The drawing under review shows one solid part. Ordinate dimensions are in mm from its lowest x, y, z. A direction names the side the tool comes from. Coordinates: 2 decimals unless noted, no trailing zeros. Write each loop counter-clockwise with the first axis right and the second up, starting at its lowest first coordinate (ties: lowest second). Pieces come first, ordered by that corner, then holes.
1) For P1, Ø2, axis at x = 31, z = 14.5, coming from the +Y side; P2, Ø3, axis at x = 23.5, y = 33, coming from the +Z side; P3, Ø1.5, axis at y = 26, z = 5.5, coming from the +X side; P4, Ø4, axis at y = 11, z = 17.5, coming from the +X side, all flat-tipped, find the tip position at first contact; note any pin that passes through.
2) Add section B-B, the plane z = 1.75. State the section outline as (x, y) points.
3) Add section A-A, the plane z = 21.5. State the section outline as (x, y) points.
4) Machinability: for the marked faces 1 and 2, which of the approach directions +Z, -Z, +X, -X, +Y, -Y give a long, thin tool a straight path to every point of the face, cutting with its end or side? Answer none if there is none.
5) For line 1 (Z direction, x = 6.5, y = 6.5); line 2 (X direction, y = 35, z = 4.75) (1 decimal); line 3 (Y direction, x = 27.5, z = 4), list the stretches that pass through material, from the lowest coordinate up.
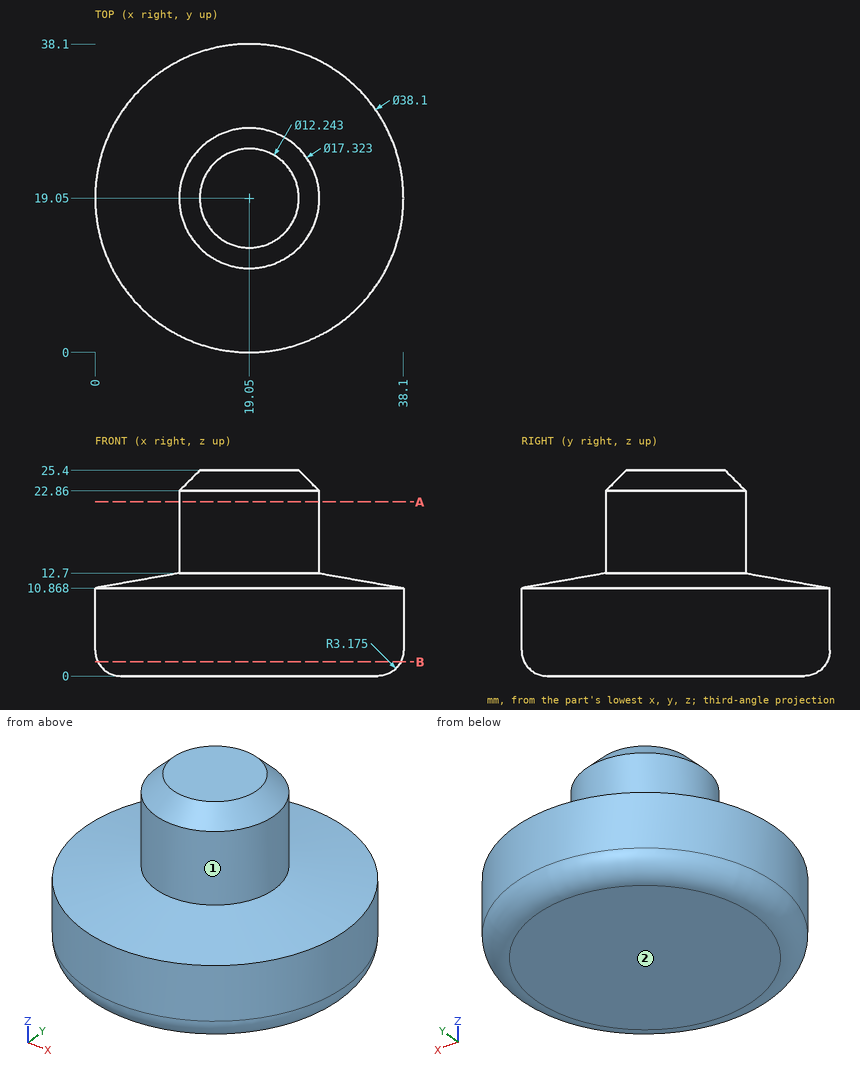
Geometry results:
1. P1: passes through
1. P2: stops at z = 11.91
1. P3: stops at x = 37.06
1. P4: stops at x = 25.25
2. outline: circle Ø37.42 at (19.05, 19.05)
3. outline: circle Ø17.32 at (19.05, 19.05)
4. face 1: +Z
4. face 2: -Z, +X, -X, +Y, -Y
5. line 1: z = 0.61 to 11.1
5. line 2: x = 8.6 to 29.5
5. line 3: y = 1.98 to 36.12
